```python
from build123d import *

# Parameters (mm, degrees)
ESBO_O1_R                 = 35
RESSALTO_EXTRUS_O1_DEPTH  = 5
ESBO_O3_R                 = 10
RESSALTO_EXTRUS_O3_DEPTH  = 13
ESBO_O4_R                 = 5
CORTE_EXTRUS_O1_DEPTH     = 13
RESSALTO_EXTRUS_O5_DEPTH  = 13
CORTE_EXTRUS_O6_START     = -11
CORTE_EXTRUS_O6_OUTLINE_R = 2
CORTE_EXTRUS_O6_DEPTH     = 22
CORTE_EXTRUS_O8_DEPTH     = 68.852738868
RESSALTO_EXTRUS_O7_DEPTH  = 26
ESBO_O19_R                = 1.5
CORTE_EXTRUS_O9_DEPTH     = 26
FILETE1_R                 = 10
FILETE2_R                 = 10
RESSALTO_EXTRUS_O9_DEPTH  = 12
CORTE_EXTRUS_O11_REACH    = 75.407
ESBO_O26_R                = 3
CHANFRO7_SIZE             = 3
CHANFRO8_SIZE             = 3
CHANFRO9_SIZE             = 3
CHANFRO10_SIZE            = 2
FILETE5_R                 = 2
FILETE6_R                 = 2
CHANFRO11_SIZE            = 2


with BuildPart() as part:
    # Esboço1 → Ressalto-extrusão1 (new body)
    with BuildSketch(Plane(origin=(0, 0, 0), x_dir=(1, 0, 0), z_dir=(0, 1, 0))):
        with Locations(Location((0, 0, 0), (0, 0, 270))):
            Circle(ESBO_O1_R)
    extrude(amount=RESSALTO_EXTRUS_O1_DEPTH)

    # Esboço3 → Ressalto-extrusão3 (add)
    with BuildSketch(Plane.XZ):
        with Locations(Location((0, 0, 0), (0, 0, 90))):
            Circle(ESBO_O3_R)
    extrude(amount=RESSALTO_EXTRUS_O3_DEPTH)

    # Esboço4 → Corte-extrusão1 (cut)
    with BuildSketch(Plane(origin=(0, -13, 0), x_dir=(-1, 0, 0), z_dir=(0, -1, 0))):
        with Locations(Location((0, 0, 0), (0, 0, 90))):
            Circle(ESBO_O4_R)
    extrude(amount=-CORTE_EXTRUS_O1_DEPTH, mode=Mode.SUBTRACT)

    # Esboço11 → Ressalto-extrusão5 (add)
    with BuildSketch(Plane.XZ):
        Polygon((10.27244843, -26.12425699), (10.703764509, -27.026457876), (14.312568056, -25.301193562), (13.449935899, -23.496791788), (9.841132351, -25.222056103), align=None)
    extrude(amount=RESSALTO_EXTRUS_O5_DEPTH)

    # Corte-extrusão6: read off the stored shape, not the designer's step
    # Corte-extrusão6 outline → Corte-extrusão6 (cut)
    with BuildSketch(Plane(origin=(0, 0, 0), x_dir=(0.9022008868624063, 0, 0.4313160786994702), z_dir=(0.43131607869947014, 0, -0.9022008868624064)).offset(CORTE_EXTRUS_O6_START)):
        with Locations((0, 7.014981428)):
            Circle(CORTE_EXTRUS_O6_OUTLINE_R)
    extrude(amount=CORTE_EXTRUS_O6_DEPTH, mode=Mode.SUBTRACT)

    # 3DSketch5 → Corte-extrusão8 (cut, through all)
    with BuildSketch(Plane(origin=(-8.247671749, -6.480100675, 16.008238046), x_dir=(0.7047714310013795, 0.6243195323179013, 0.3369307816312202), z_dir=(-0.43131607869947175, 0, 0.9022008868624055))):
        Polygon((0, 0), (-30.606987597, 24.461465293), (-10.703733889, 49.365069068), (51.063459474, 0), (31.160205765, -24.903603774), align=None)
    extrude(amount=CORTE_EXTRUS_O8_DEPTH, mode=Mode.SUBTRACT)

    # Esboço18 → Ressalto-extrusão7 (add)
    with BuildSketch(Plane(origin=(0, 5, 0), x_dir=(1, 0, 0), z_dir=(0, 1, 0))):
        Polygon((4.313160787, 9.022008869), (31.379187393, -3.917473492), (33.535767786, 0.593530942), (-20.596285425, 26.472495664), (-22.752865819, 21.96149123), align=None)
    extrude(amount=RESSALTO_EXTRUS_O7_DEPTH)

    # Esboço19 → Corte-extrusão9 (cut)
    with BuildSketch(Plane(origin=(4.313160787, 0, -9.022008869), x_dir=(0.9022008868624055, 0, 0.43131607869947175), z_dir=(-0.43131607869947175, 0, 0.9022008868624055))):
        with Locations((-22.5, 17.5)):
            Circle(ESBO_O19_R)
        with Locations((22.5, 17.5)):
            Circle(ESBO_O19_R)
    extrude(amount=-CORTE_EXTRUS_O9_DEPTH, mode=Mode.SUBTRACT)

    # Filete1
    filete1_edges = [part.edges().sort_by_distance(p)[0] for p in [
        (32.45747759, 31, 1.661971275),
        (-21.674575622, 31, -24.216993447),
    ]]
    fillet(filete1_edges, radius=FILETE1_R)

    # Filete2
    filete2_edges = [part.edges().sort_by_distance(p)[0] for p in [
        (19.317369696, 2.5, 29.18628493),
        (-34.844748529, 2.5, 3.292946997),
    ]]
    fillet(filete2_edges, radius=FILETE2_R)

    # Esboço25 → Ressalto-extrusão9 (add)
    with BuildSketch(Plane(origin=(0, 5, 0), x_dir=(1, 0, 0), z_dir=(0, 1, 0))):
        Polygon((8.981926733, 18.787851102), (-0.040082135, 23.101011889), (1.253866101, 25.80761455), (19.297883838, 17.181292976), (18.003935602, 14.474690315), align=None)
    extrude(amount=RESSALTO_EXTRUS_O9_DEPTH)

    # Esboço26 → Corte-extrusão11 (cut, up to next)
    with BuildSketch(Plane(origin=(10.275874969, 0, -21.494453763), x_dir=(-0.902200886862406, 0, -0.4313160786994711), z_dir=(0.4313160786994711, 0, -0.902200886862406)), mode=Mode.PRIVATE) as corte_extrus_o11_sk1:
        with Locations((0, 11)):
            Circle(ESBO_O26_R)
    corte_extrus_o11_tool1 = extrude(corte_extrus_o11_sk1.sketch, amount=-CORTE_EXTRUS_O11_REACH, mode=Mode.PRIVATE) & part.part
    add(corte_extrus_o11_tool1.solids().sort_by_distance((10.275875, 11, -21.494454))[0], mode=Mode.SUBTRACT)

    # Chanfro7
    chanfro7_edges = [part.edges().sort_by_distance(p)[0] for p in [
        (6.46974118, 5, -13.533013303),
    ]]
    chamfer(chanfro7_edges, length=CHANFRO7_SIZE)

    # Chanfro8
    # the kernel refuses this chamfer: 3 mm, written as the material it adds along each edge
    with BuildSketch(Plane(origin=(38.157340689, 5, -10.26065762), x_dir=(0.9022008868624055, 0, 0.43131607869947186), z_dir=(-0.4313160786994719, 0, 0.9022008868624055))) as chanfro8_piece_1_section:
        Polygon((CHANFRO8_SIZE, 0), (0, CHANFRO8_SIZE), (0, 0), align=None)
    chanfro8_piece_1 = extrude(amount=15.715048964, mode=Mode.PRIVATE)
    chanfro8_piece_1 = split(chanfro8_piece_1, bisect_by=Plane(origin=(36.493528356, 1.142475518, -6.780395611), z_dir=(-0.30498652408318644, -0.7071067811865479, 0.6379523650929244)), keep=Keep.TOP, mode=Mode.PRIVATE)
    chanfro8_piece_1 = chanfro8_piece_1 & Plane(origin=(0, 5, 0), x_dir=(0, 0, 1), z_dir=(0, -1, 0)) * Cylinder(35, 44, mode=Mode.PRIVATE)
    chanfro8_piece_1 = split(chanfro8_piece_1, bisect_by=Plane(origin=(33.535767786, 5, -0.593530942), z_dir=(0.4313160786994711, 0, -0.9022008868624058)), keep=Keep.TOP, mode=Mode.PRIVATE)
    add(chanfro8_piece_1)
    with BuildSketch(Plane(origin=(38.157340689, 5, -10.26065762), x_dir=(0.9022008868624055, 0, 0.43131607869947186), z_dir=(-0.4313160786994719, 0, 0.9022008868624055))) as chanfro8_piece_2_section:
        Polygon((CHANFRO8_SIZE, 0), (0, CHANFRO8_SIZE), (0, 0), align=None)
    chanfro8_piece_2 = extrude(amount=15.715048964, mode=Mode.PRIVATE)
    chanfro8_piece_2 = split(chanfro8_piece_2, bisect_by=Plane(origin=(36.493528356, 1.142475518, -6.780395611), z_dir=(-0.30498652408318644, -0.7071067811865479, 0.6379523650929244)), keep=Keep.TOP, mode=Mode.PRIVATE)
    chanfro8_piece_2 = chanfro8_piece_2 & Plane(origin=(0, 5, 0), x_dir=(0, 0, 1), z_dir=(0, -1, 0)) * Cylinder(35, 44, mode=Mode.PRIVATE)
    chanfro8_piece_2 = split(chanfro8_piece_2, bisect_by=Plane(origin=(33.535767786, 5, -0.593530942), z_dir=(-0.4313160786994711, 0, 0.9022008868624058)), keep=Keep.TOP, mode=Mode.PRIVATE)
    add(chanfro8_piece_2)

    # Chanfro9
    # the kernel refuses this chamfer: 3 mm, written as the material it adds along each edge
    with BuildSketch(Plane(origin=(-22.752865819, 5, -21.96149123), x_dir=(0, 1, 0), z_dir=(0.431316078699471, 0, -0.902200886862406))) as chanfro9_piece_1_section:
        Polygon((CHANFRO9_SIZE, 0), (0, -CHANFRO9_SIZE), (0, 0), align=None)
    chanfro9_piece_1 = extrude(amount=15.715048964, mode=Mode.PRIVATE)
    chanfro9_piece_1 = split(chanfro9_piece_1, bisect_by=Plane(origin=(-20.596285425, 5, -26.472495664), z_dir=(-0.4313160786994711, 0, 0.9022008868624058)), keep=Keep.TOP, mode=Mode.PRIVATE)
    chanfro9_piece_1 = split(chanfro9_piece_1, bisect_by=Plane(origin=(-21.027601504, 9, -25.570294777), z_dir=(-0.30498652408290505, -0.7071067811867798, 0.6379523650928014)), keep=Keep.TOP, mode=Mode.PRIVATE)
    chanfro9_piece_1 = chanfro9_piece_1 & Plane(origin=(0, 5, 0), x_dir=(0, 0, 1), z_dir=(0, -1, 0)) * Cylinder(35, 44, mode=Mode.PRIVATE)
    add(chanfro9_piece_1)
    with BuildSketch(Plane(origin=(-22.752865819, 5, -21.96149123), x_dir=(0, 1, 0), z_dir=(0.431316078699471, 0, -0.902200886862406))) as chanfro9_piece_2_section:
        Polygon((CHANFRO9_SIZE, 0), (0, -CHANFRO9_SIZE), (0, 0), align=None)
    chanfro9_piece_2 = extrude(amount=15.715048964, mode=Mode.PRIVATE)
    chanfro9_piece_2 = split(chanfro9_piece_2, bisect_by=Plane(origin=(-20.596285425, 5, -26.472495664), z_dir=(0.4313160786994711, 0, -0.9022008868624058)), keep=Keep.TOP, mode=Mode.PRIVATE)
    chanfro9_piece_2 = split(chanfro9_piece_2, bisect_by=Plane(origin=(-21.027601504, 9, -25.570294777), z_dir=(-0.30498652408290505, -0.7071067811867798, 0.6379523650928014)), keep=Keep.TOP, mode=Mode.PRIVATE)
    chanfro9_piece_2 = chanfro9_piece_2 & Plane(origin=(0, 5, 0), x_dir=(0, 0, 1), z_dir=(0, -1, 0)) * Cylinder(35, 44, mode=Mode.PRIVATE)
    add(chanfro9_piece_2)

    # Chanfro10
    chanfro10_edges = [part.edges().sort_by_distance(p)[0] for p in [
        (18.65090972, 5, -15.827991645),
        (10.275874969, 5, -21.494453763),
        (0.606891983, 5, -24.454313219),
        (8.981926733, 5, -18.787851102),
    ]]
    chamfer(chanfro10_edges, length=CHANFRO10_SIZE)

    # Filete5
    filete5_edges = [part.edges().sort_by_distance(p)[0] for p in [
        (10.275874969, 17, -21.494453763),
    ]]
    fillet(filete5_edges, radius=FILETE5_R)

    # Filete6
    # the kernel refuses this fillet: 2 mm, written as the material it takes off along each edge
    with BuildSketch(Plane(origin=(21.910580039, 17, -12.607036909), x_dir=(0.4313160786994712, -7.105427357600661e-14, -0.9022008868624057), z_dir=(-0.9022008868624058, 0, -0.4313160786994713))) as filete6_piece_1:
        with BuildLine():
            CenterArc((2, 1.732050808), FILETE6_R, 180, 60)
            Line((0, 1.732050808), (-0.04, 1.732050808))
            Line((-0.04, 1.732050808), (-0.04, 0))
            Line((-0.04, 0), (0, -0.04))
            ThreePointArc((0, -0.04), (0.5, -0.04), (0.98, -0.034641016))
            Line((0.98, -0.034641016), (1, 0))
        make_face()
    extrude(amount=28.660254038, mode=Mode.SUBTRACT)

    # Chanfro11
    chanfro11_edges = [part.edges().sort_by_distance(p)[0] for p in [
        (10.27244843, 0, -26.12425699),
        (12.508166282, 0, -26.163825719),
        (13.881251977, 0, -24.398992675),
        (11.645534125, 0, -24.359423945),
    ]]
    chamfer(chanfro11_edges, length=CHANFRO11_SIZE)


solid = part.part
```
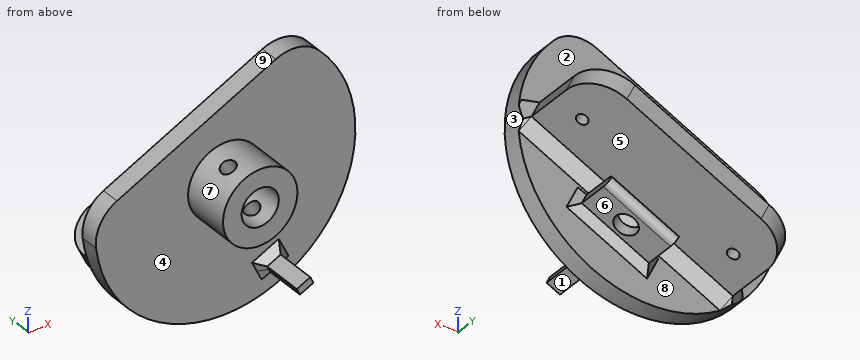
For this review, take the finished solid that the model builds, in its own axes (mm). Face numbers are marked on the shaded views. A direction names the side the tool comes from. Round coordinates to 2 decimals unless told otherwise and drop trailing zeros. Write each loop counter-clockwise with the first axis right and the second up, starting at its lowest first coordinate (ties: lowest second). Pieces come first, ordered by that corner, then holes. Notation, with made-up numbers: (44.5, 11.25) -> (80.5, 11.25) arc R11 cw to (80.5, 25.25) -> close; hole circle Ø1 at (76, 31.25). An arc over 180 degrees is marked (long way). Use one line per item in the form item = value.
1) Tool access review of the marked faces 1, 2, 3, 4 and 5: name each direction out of +Z, -Z, +X, -X, +Y, -Y from which nothing blocks a thin tool from reaching the whole face with its end or side.
Found:
face_1 = -Z, +X, -Y
face_2 = +Z, -X, +Y
face_3 = +Y, -Y
face_4 = -Y
face_5 = +Y
2) Clearance check with flat-ended pins moving along their axes: pin 1 (5 mm diameter, centred on x = 6.5, z = -21, fed in from +Y); pin 2 (10 mm diameter, centred on x = -20, y = -1.5, fed in from +Z); pin 3 (8 mm diameter, centred on x = 10.5, y = 14.5, fed in from +Z); pin 4 (10 mm diameter, centred on x = -24, y = -8.5, fed in from +Z). State where each tip first meets the part, or that it passes through.
Found:
pin_1 = 17
pin_2 = 12.67
pin_3 = -4.15
pin_4 = through
3) Take a section at A-A, the plane y = -4. Write out the cut boundary in (x, z).
Found:
outline = circle Ø20 at (0, 0); (9.84, -25.22) -> (10.7, -27.03) -> (14.31, -25.3) -> (13.45, -23.5) -> close; hole circle Ø10 at (0, 0)
4) Mouldability with a two-part tool opening along X and no side actions: class the marked faces 6, 7, 8 and 9 as +X half, -X half, draft (parallel to the pull), parting line (faces both ways), or undercut.
Found:
face_6 = +X half
face_7 = parting line
face_8 = undercut
face_9 = -X half
5) To check wall thickness, follow L1, parallel to X at y = -3, z = 0; L2, parallel to Y at x = -21.5, z = -2; L3, parallel to Y at x = -7.5, z = -15. State the ranges of each line that lie inside material, in increasing order. Write a range as from..to.
Found:
L1 = -10..-5, 5..10
L2 = 0..5
L3 = 0..31
6) Take a section at B-B, the plane y = 9. Write out the cut boundary in (x, z), and give its area (3 significant figures).
Found:
outline = (-22.75, -21.96) -> (-20.6, -26.47) -> (33.54, -0.59) -> (31.38, 3.92) -> close; (-0.04, -23.1) -> (1.25, -25.81) -> (8.26, -22.46) -> (6.96, -19.75) -> close; (11, -17.82) -> (12.29, -20.53) -> (19.3, -17.18) -> (18, -14.47) -> close
area = 347 mm2
